For this review, take the finished solid that the model builds, in its own axes (mm). Coordinates: 2 decimals unless noted, no trailing zeros. Loops run counter-clockwise (first coordinate to the right, second up) from the corner with the lowest first, then second, coordinate; pieces in that order, holes last. Notation, with made-up numbers: M 79,74.5 L 116,74.5 A23 cw 116,101.5 Z; hole C 19.25,-3 d11. An arc over 180 degrees is marked long. Write item = value, one per line.
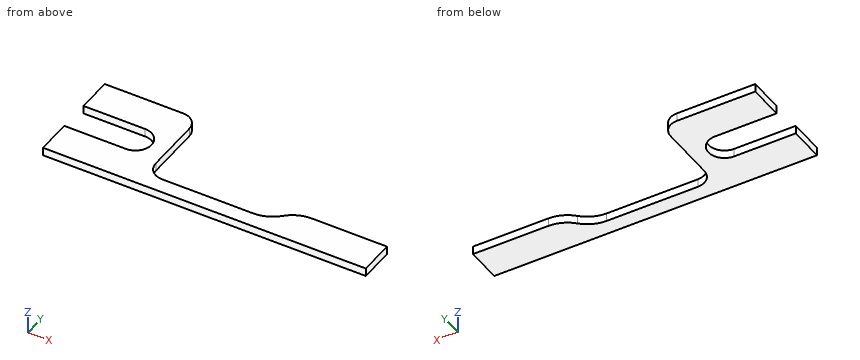
Autodesk Inventor part; units mm, degrees
ref_plane "YZ Plane" through (0, 0, 0) normal (1, 0, 0) x (0, 1, 0)
ref_plane "XZ Plane" through (0, 0, 0) normal (0, 1, 0) x (-1, 0, 0)
ref_plane "XY Plane" through (0, 0, 0) normal (0, 0, 1) x (1, 0, 0)
sketch "Sketch1" plane through (0, 0, 0) normal (0, 0, 1) x (1, 0, 0)
  line L0 (-15.24, 5.08) -> (15.24, 5.08)
  line L1 (15.24, 5.08) -> (15.24, -5.08)
  line L2 (15.24, -5.08) -> (-15.24, -5.08)
  line L3 (-15.24, -5.08) -> (-15.24, 5.08)
  point P0 (0, 0)
  point P1 (0, 5.08)
  point P2 (-15.24, 0)
  dimension "d0" = 30.48
  dimension "d1" = 10.16
extrude "Extrusion1" add sketch "Sketch1" along normal blind 0.8128
sketch "Sketch2" plane through (0, 0, 0.8128) normal (0, 0, 1) x (1, 0, 0)
  line L0 (15.24, 5.08) -> (15.24, -5.08)
  line L1 (-15.24, 5.08) -> (15.24, 5.08)
  line L2 (-15.24, -5.08) -> (-15.24, 5.08)
  line L3 (15.24, -5.08) -> (-15.24, -5.08)
  line L4 (-4.3525, 3.556) -> (2.3785, 3.556)
  line L5 (-4.3525, -3.556) -> (2.3785, -3.556)
  line L6 (-5.94, 1.9685) -> (-5.94, -1.9685)
  line L7 (3.966, 1.9685) -> (3.966, -1.9685)
  arc A0 (-4.3525, 3.556) -> (-5.94, 1.9685) centre (-4.3525, 1.9685) ccw
  arc A1 (-5.94, -1.9685) -> (-4.3525, -3.556) centre (-4.3525, -1.9685) ccw
  arc A2 (2.3785, -3.556) -> (3.966, -1.9685) centre (2.3785, -1.9685) ccw
  arc A3 (3.966, 1.9685) -> (2.3785, 3.556) centre (2.3785, 1.9685) ccw
  point P0 (-0.987, 3.556)
  point P1 (-0.987, -3.556)
  point P2 (-5.94, 0)
  point P3 (3.966, 0)
  dimension "d5" = 6.731
  dimension "d6" = 6.731
  dimension "d7" = 3.937
  dimension "d8" = 3.937
  dimension "d13" = 1.5875
  dimension "d14" = 1.5875
  dimension "d15" = 1.5875
  dimension "d16" = 1.5875
  dimension "d38" = 9.3
extrude "Extrusion2" cut sketch "Sketch2" against normal blind 25.4 contours L4 A3 L7 A2 L5 A1 L6 A0
sketch "Sketch3" plane through (0, 0, 0.8128) normal (0, 0, 1) x (1, 0, 0)
  arc A0 (-4.3525, 3.556) -> (-5.94, 1.9685) centre (-4.3525, 1.9685) ccw
  line L0 (-4.3525, 3.556) -> (2.3785, 3.556)
  arc A1 (3.966, 1.9685) -> (2.3785, 3.556) centre (2.3785, 1.9685) ccw
  line L1 (3.966, 1.9685) -> (3.966, -1.9685)
  arc A2 (2.3785, -3.556) -> (3.966, -1.9685) centre (2.3785, -1.9685) ccw
  line L2 (2.3785, -3.556) -> (-4.3525, -3.556)
  arc A3 (-5.94, -1.9685) -> (-4.3525, -3.556) centre (-4.3525, -1.9685) ccw
  line L3 (-5.94, -1.9685) -> (-5.94, 1.9685)
  line L4 (15.24, 5.08) -> (15.24, -5.08)
  line L5 (-15.24, 5.08) -> (15.24, 5.08)
  line L6 (-15.24, -5.08) -> (-15.24, 5.08)
  line L7 (15.24, -5.08) -> (-15.24, -5.08)
  line L8 (-15.24, 1.5875) -> (-9.13, 1.5875)
  line L9 (-15.24, -1.5875) -> (-9.13, -1.5875)
  arc A4 (-9.13, -1.5875) -> (-9.13, 1.5875) centre (-9.13, 0) ccw
  point P0 (0, 0)
  dimension "d20" = 3.4925
  dimension "d21" = 6.11
  dimension "d22" = 3.175
  dimension "d24" = 1.5875
extrude "Extrusion3" cut sketch "Sketch3" against normal blind 25.4 contours L8 A4 L9 L6
mirror "Mirror1" about plane through (0, 0, 0) normal (1, 0, 0) of "Extrusion3"
sketch "Sketch5" plane through (0, 0, 0.8128) normal (0, 0, 1) x (1, 0, 0)
  line L0 (3.966, 1.9685) -> (3.966, -1.9685) construction
  line L1 (-5.94, -1.9685) -> (3.966, -1.9685)
  line L2 (3.966, -1.9685) -> (3.966, 7.0011)
  line L3 (3.966, 7.0011) -> (-5.94, 7.0011)
  line L4 (-5.94, 7.0011) -> (-5.94, -1.9685)
  point P0 (0, 0)
extrude "Extrusion5" cut sketch "Sketch5" against normal through all
fillet "Fillet1" radius 1.524 2 edges at (-5.94, 5.08, 0.4064) (3.966, 5.08, 0.4064)
sketch "Sketch7" plane through (0, 0, 0.8128) normal (0, 0, 1) x (1, 0, 0)
  line L0 (9.13, -1.5875) -> (15.24, -1.5875) construction
  line L1 (15.24, -1.5875) -> (3.966, -1.5875)
  line L2 (3.966, -1.5875) -> (3.966, 5.08)
  line L3 (3.966, 5.08) -> (15.24, 5.08)
  line L4 (15.24, 5.08) -> (15.24, -1.5875)
  line L5 (3.966, 3.556) -> (3.966, -1.9685)
  point P0 (0, 0)
extrude "Extrusion6" cut sketch "Sketch7" against normal through all
sketch "Sketch8" plane through (0, 0, 0.8128) normal (0, 0, 1) x (1, 0, 0)
  line L0 (3.966, -1.5875) -> (15.24, -1.5875)
  arc A0 (2.3785, -3.556) -> (3.966, -1.9685) centre (2.3785, -1.9685) ccw
  line L1 (7.62, -1.5875) -> (2.3785, -1.5875)
  line L2 (2.3785, -1.5875) -> (2.3785, -3.556)
  line L3 (2.3785, -3.556) -> (7.62, -3.556)
  line L4 (7.62, -3.556) -> (7.62, -1.5875)
  line L5 (15.24, -1.5875) -> (15.24, -5.08)
  point P0 (0, 0)
  dimension "d34" = 7.62
extrude "Extrusion7" cut sketch "Sketch8" against normal through all
fillet "Fillet2" radius 3.175 2 edges at (7.62, -3.556, 0.4064) (7.62, -1.5875, 0.4064)
sketch "Sketch9" plane through (15.24, -5.08, 0.8128) normal (1, 0, 0) x (0, 0, -1)
  line L0 (0.8128, 3.4925) -> (0, 3.4925)
  line L1 (0, 3.4925) -> (0, 0)
  line L2 (0.8128, 0) -> (0, 0)
  line L3 (0.8128, 3.4925) -> (0.8128, 0)
  point P0 (0.8128, 5.08)
extrude "Extrusion8" add sketch "Sketch9" along normal blind 1.5
properties part number "HarveyHeadplate_LargerCenter_FrontAndSideCutout_WiderTeeth_Ver3"
Q1. Add section A-A (x = -10). Write out the cut boundary in (y, z).
Solved:
outline = M -5.08,0 L -1.59,0 L -1.59,0.81 L -5.08,0.81 Z; M 1.59,0 L 5.08,0 L 5.08,0.81 L 1.59,0.81 Z
Q2. Add section B-B (y = -2.25). Write out the cut boundary in (x, z).
Solved:
outline = M -15.24,0 L -5.91,0 L -5.91,0.81 L -15.24,0.81 Z; M 7.34,0 L 16.74,0 L 16.74,0.81 L 7.34,0.81 Z
Q3. For line 1 along Y through (x, z) = (-9.5, 0.45); line 2 along Y through (x, z) = (-3, 0.15); line 3 along X through (y, z) = (-3.25, 0.65), list the stretches that pass through material, from the lowest coordinate up.
Solved:
line_1 = -5.08 to -1.59, 1.59 to 5.08
line_2 = -5.08 to -3.56
line_3 = -15.24 to -5.29, 6.04 to 16.74
Q4. Add section D-D (y = 0). Write out the cut boundary in (x, z), and give its area (3 significant figures).
Solved:
outline = M -7.54,0 L -5.94,0 L -5.94,0.81 L -7.54,0.81 Z
area = 1.30 mm²
